Check sheet for the modelled part. Datum: model origin and axes. Units: mm. A direction names the side the tool comes from. Give positions to 0.01 mm unless a question says otherwise; leave off trailing zeros. Order: outer loops, then holes, each group sorted by start corner. A loop starts at its lowest first (then second) coordinate and runs counter-clockwise, first axis right, second up. Notation, with made-up numbers: (-37.5, 74.5) -> (-32.5, 74.5) arc R26 ccw to (-32.5, 101.5) -> close; hole circle Ø1 at (67, 28.25). An arc over 180 degrees is marked (long way). Answer in a Markdown table with one row per item. Add a question column.
(1) Set-up check for faces 1 (the face through (52, -5, 0)), 2 (the face through (-71.85, 35.94, -14.93)), 3 (the face through (-71.373, 18, 0)): record each of +Z, -Z, +X, -X, +Y, -Y from which the full face is reachable in a straight line by a thin tool's end or side.
(2) Cross-section at A-A (z = -15.5). Record the cut outline in (x, y).
(3) Cross-section at D-D (x = -4). Record the cut outline in (y, z), then the cut area to 3 significant figures.
(4) Cross-section at C-C (z = -8). Record the cut outline in (x, y).
(5) Thickness scan on L1, parallel to X at y = 23, z = -9.25; L2, parallel to X at y = 32, z = -5.25; L3, parallel to X at y = 13.5, z = 5.25. Record the ranges inside material, lowest first. Write a range as [from, to].
(6) Go/stop test with flat-tipped pins: pin 1 (6.5 mm diameter, centred on x = 65.5, y = 47.5, fed in from -Z); pin 2 (16 mm diameter, centred on x = 3, z = 0, fed in from +Y); pin 3 (14.5 mm diameter, centred on x = -49, z = 5, fed in from +Y). Record where each tip stops, or that it passes through.
(7) Release check for a two-part mould opening along X. For faces 4 (the face through (27.594, 10.389, -14.93)), 5 (the face through (22.879, 18.752, -14.93)), 6 (the face through (6, -6, 10)), 7 (the face through (-20.279, 23.255, 0.14)) record: released by +X, released by -X, zero draft, split by the parting line, or undercut.
(8) Cross-section at B-B (y = -1.5). Record the cut outline in (x, z), then the cut area to 3 significant figures.
```python
from build123d import *

# Parameters (mm, degrees)
BOSS_EXTRU_1_DEPTH      = 10
ESQUISSE2_R             = 6.5
ENL_V_MAT_EXTRU_1_DEPTH = 63
ESQUISSE3_R             = 6.5
ENL_V_MAT_EXTRU_2_DEPTH = 63
CONG_1_R                = 10
CONG_2_R                = 10
BOSS_EXTRU_2_START      = -2
ESQUISSE4_R             = 6.5
ESQUISSE4_R_2           = 5.7
BOSS_EXTRU_2_DEPTH      = 2
BOSS_EXTRU_3_START      = -2
ESQUISSE5_R             = 6.5
ESQUISSE5_R_2           = 5.7
BOSS_EXTRU_3_DEPTH      = 2
BOSS_EXTRU_4_START      = -2
ESQUISSE6_R             = 6.5
ESQUISSE6_R_2           = 5.7
BOSS_EXTRU_4_DEPTH      = 2
BOSS_EXTRU_5_START      = -2
ESQUISSE7_R             = 6.5
ESQUISSE7_R_2           = 5.7
BOSS_EXTRU_5_DEPTH      = 2
BOSS_EXTRU_6_DEPTH      = 10


with BuildPart() as part:
    # Esquisse1 → Boss.-Extru.1 (new, symmetric)
    with BuildSketch(Plane.XY):
        Polygon((23.267949192, 24.980762114), (33.267949192, 7.660254038), (33.267949192, -5), (71.373066959, -5), (71.373066959, 29.660254038), (61.373066959, 46.980762114), (67.435244785, 50.480762114), (77.435244785, 33.160254038), (77.435244785, -15), (71.373066959, -15), (-71.373066959, -15), (-77.435244785, -15), (-77.435244785, 33.160254038), (-67.435244785, 50.480762114), (-61.373066959, 46.980762114), (-71.373066959, 29.660254038), (-71.373066959, -5), (-33.267949192, -5), (-33.267949192, 7.660254038), (-23.267949192, 24.980762114), (-17.205771366, 21.480762114), (-27.205771366, 4.160254038), (-27.205771366, -5), (27.205771366, -5), (27.205771366, 4.160254038), (17.205771366, 21.480762114), align=None)
    extrude(amount=BOSS_EXTRU_1_DEPTH, both=True)

    # Esquisse2 → Enlèv. mat.-Extru.1 (cut)
    with BuildSketch(Plane(origin=(-72.435244785, 41.820508076, 0), x_dir=(0, 0, 1), z_dir=(-0.8660254037844399, 0.4999999999999977, 0))):
        with Locations(Location((0, 0, 0), (0, 0, 270))):
            Circle(ESQUISSE2_R)
    extrude(amount=-ENL_V_MAT_EXTRU_1_DEPTH, mode=Mode.SUBTRACT)

    # Esquisse3 → Enlèv. mat.-Extru.2 (cut)
    with BuildSketch(Plane(origin=(72.435244785, 41.820508076, 0), x_dir=(0, 0, -1), z_dir=(0.86602540378444, 0.4999999999999975, 0))):
        with Locations(Location((0, 0, 0), (0, 0, 90))):
            Circle(ESQUISSE3_R)
    extrude(amount=-ENL_V_MAT_EXTRU_2_DEPTH, mode=Mode.SUBTRACT)

    # Congé1
    cong_1_edges = [part.edges().sort_by_distance(p)[0] for p in [
        (33.267949192, -5, 0),
        (71.373066959, -5, 0),
        (-71.373066959, -5, 0),
        (-33.267949192, -5, 0),
    ]]
    fillet(cong_1_edges, radius=CONG_1_R)

    # Congé2
    # the kernel refuses this fillet: 10 mm, written as the material it adds along each edge
    with BuildSketch(Plane(origin=(-27.205771366, -5, 10), x_dir=(1, 0, 0), z_dir=(0, 0, -1))) as cong_2_piece_1:
        with BuildLine():
            CenterArc((9.964678957, -10), CONG_2_R, 90, 85.182937258)
            Line((0, -9.160254038), (-0.199293579, -9.143459119))
            ThreePointArc((-0.199293579, -9.143459119), (-0.2, -4.580127019), (-0.2, 0))
            Line((-0.2, 0), (0, 0.2))
            Line((0, 0.2), (9.964678957, 0.2))
            Line((9.964678957, 0.2), (9.964678957, 0))
        make_face()
    extrude(amount=20)
    with BuildSketch(Plane(origin=(27.205771366, -5, 10), x_dir=(0, 1, 0), z_dir=(0, 0, -1))) as cong_2_piece_2:
        with BuildLine():
            CenterArc((10, -9.964678957), CONG_2_R, 94.817062742, 85.182937258)
            Line((0, -9.964678957), (-0.2, -9.964678957))
            Line((-0.2, -9.964678957), (-0.2, 0))
            Line((-0.2, 0), (0, 0.2))
            ThreePointArc((0, 0.2), (4.580127019, 0.2), (9.143459119, 0.199293579))
            Line((9.143459119, 0.199293579), (9.160254038, 0))
        make_face()
    extrude(amount=20)

    # Esquisse4 → Boss.-Extru.2 (add)
    with BuildSketch(Plane(origin=(-22.205771366, 12.820508076, 0), x_dir=(0, 0, -1), z_dir=(0.8660254037844398, -0.49999999999999817, 0)).offset(BOSS_EXTRU_2_START)):
        with Locations(Location((0, 0, 0), (0, 0, 90))):
            Circle(ESQUISSE4_R)
        with Locations(Location((0, 0, 0), (0, 0, 90))):
            Circle(ESQUISSE4_R_2, mode=Mode.SUBTRACT)
    extrude(amount=BOSS_EXTRU_2_DEPTH)

    # Esquisse5 → Boss.-Extru.3 (add)
    with BuildSketch(Plane(origin=(-66.373066959, 38.320508076, 0), x_dir=(0, 0, -1), z_dir=(0.8660254037844398, -0.49999999999999817, 0)).offset(BOSS_EXTRU_3_START)):
        with Locations(Location((0, 0, 0), (0, 0, 270))):
            Circle(ESQUISSE5_R)
        with Locations(Location((0, 0, 0), (0, 0, 90))):
            Circle(ESQUISSE5_R_2, mode=Mode.SUBTRACT)
    extrude(amount=BOSS_EXTRU_3_DEPTH)

    # Esquisse6 → Boss.-Extru.4 (add)
    with BuildSketch(Plane(origin=(22.205771366, 12.820508076, 0), x_dir=(0, 0, 1), z_dir=(-0.8660254037844398, -0.49999999999999817, 0)).offset(BOSS_EXTRU_4_START)):
        with Locations(Location((0, 0, 0), (0, 0, 270))):
            Circle(ESQUISSE6_R)
        with Locations(Location((0, 0, 0), (0, 0, 270))):
            Circle(ESQUISSE6_R_2, mode=Mode.SUBTRACT)
    extrude(amount=BOSS_EXTRU_4_DEPTH)

    # Esquisse7 → Boss.-Extru.5 (add)
    with BuildSketch(Plane(origin=(66.373066959, 38.320508076, 0), x_dir=(0, 0, 1), z_dir=(-0.8660254037844398, -0.49999999999999817, 0)).offset(BOSS_EXTRU_5_START)):
        with Locations(Location((0, 0, 0), (0, 0, 90))):
            Circle(ESQUISSE7_R)
        with Locations(Location((0, 0, 0), (0, 0, 270))):
            Circle(ESQUISSE7_R_2, mode=Mode.SUBTRACT)
    extrude(amount=BOSS_EXTRU_5_DEPTH)

    # Esquisse8 → Boss.-Extru.6 (add)
    with BuildSketch(Plane(origin=(0, 0, -10), x_dir=(-1, 0, 0), z_dir=(0, 0, -1))):
        Polygon((63.973066959, 42.477430014), (70.035244785, 45.977430014), (74.835244785, 37.663586138), (68.773066959, 34.163586138), align=None)
        Polygon((19.805771366, 16.977430014), (25.867949192, 20.477430014), (30.667949192, 12.163586138), (24.605771366, 8.663586138), align=None)
        Polygon((-25.867949192, 20.477430014), (-19.805771366, 16.977430014), (-24.605771366, 8.663586138), (-30.667949192, 12.163586138), align=None)
        Polygon((-70.035244785, 45.977430014), (-63.973066959, 42.477430014), (-68.773066959, 34.163586138), (-74.835244785, 37.663586138), align=None)
    extrude(amount=BOSS_EXTRU_6_DEPTH)


solid = part.part
```
Answer below:
| question | item | result |
|---|---|---|
| 1 | face 1 | +Z, -Z, +Y |
| 1 | face 2 | -Z, -X, -Y |
| 1 | face 3 | +Z, -Z |
| 2 | outline | (-74.84, 37.66) -> (-68.77, 34.16) -> (-63.97, 42.48) -> (-70.04, 45.98) -> close; (-30.67, 12.16) -> (-24.61, 8.66) -> (-19.81, 16.98) -> (-25.87, 20.48) -> close; (19.81, 16.98) -> (24.61, 8.66) -> (30.67, 12.16) -> (25.87, 20.48) -> close; (63.97, 42.48) -> (68.77, 34.16) -> (74.84, 37.66) -> (70.04, 45.98) -> close |
| 3 | outline | (-15, -10) -> (-5, -10) -> (-5, 10) -> (-15, 10) -> close |
| 3 | area | 200 mm² |
| 4 | outline | (-77.44, -15) -> (77.44, -15) -> (77.44, 33.16) -> (67.44, 50.48) -> (61.37, 46.98) -> (71.37, 29.66) -> (71.37, 5) arc R10 cw to (61.37, -5) -> (43.27, -5) arc R10 cw to (33.27, 5) -> (33.27, 7.66) -> (23.27, 24.98) -> (17.21, 21.48) -> (27.21, 4.16) arc R10 cw to (17.24, -5) -> (-17.24, -5) arc R10 cw to (-27.21, 4.16) -> (-17.21, 21.48) -> (-23.27, 24.98) -> (-33.27, 7.66) -> (-33.27, 5) arc R10 cw to (-43.27, -5) -> (-61.37, -5) arc R10 cw to (-71.37, 5) -> (-71.37, 29.66) -> (-61.37, 46.98) -> (-67.44, 50.48) -> (-77.44, 33.16) -> close |
| 5 | L1 | x = [-77.44, -71.37], [-24.41, -19.84], [19.84, 24.41], [71.37, 77.44] |
| 5 | L2 | x = [-77.44, -70.02], [70.02, 77.44] |
| 5 | L3 | x = [-77.44, -71.37], [71.37, 77.44] |
| 6 | pin 1 | stops at z = -10 |
| 6 | pin 2 | stops at y = -5 |
| 6 | pin 3 | stops at y = -4.88 |
| 7 | face 4 | released by +X |
| 7 | face 5 | undercut |
| 7 | face 6 | zero draft |
| 7 | face 7 | undercut |
| 8 | outline | (-77.44, -10) -> (-68.97, -10) -> (-68.97, 10) -> (-77.44, 10) -> close; (-35.67, -10) -> (-24.84, -10) -> (-24.84, 10) -> (-35.67, 10) -> close; (24.84, -10) -> (35.67, -10) -> (35.67, 10) -> (24.84, 10) -> close; (68.97, -10) -> (77.44, -10) -> (77.44, 10) -> (68.97, 10) -> close |
| 8 | area | 772 mm² |
